from build123d import *

# Parameters (mm, degrees)
SKETCH1_W               = 25.4
SKETCH1_H               = 25.4
BOSS_EXTRUDE1_DEPTH     = 5
F_1_4_CLEARANCE_HOLE1_D = 6.7564
SKETCH4_R               = 1.75
SKETCH4_W               = 25.4
SKETCH4_H               = 5
BOSS_EXTRUDE2_DEPTH     = 3
FILLET1_R               = 6


with BuildPart() as part:
    # Sketch1 → Boss-Extrude1 (new body)
    with BuildSketch(Plane(origin=(0, 0, 0), x_dir=(1, 0, 0), z_dir=(0, 1, 0))):
        Rectangle(SKETCH1_W, SKETCH1_H)
    extrude(amount=BOSS_EXTRUDE1_DEPTH)

    # 1/4 Clearance Hole1 (through all)
    with Locations(Plane(origin=(0, 5, 0), x_dir=(1, 0, 0), z_dir=(0, 1, 0))):
        with Locations((0, 0)):
            Hole(F_1_4_CLEARANCE_HOLE1_D / 2)

    # Sketch4 → Boss-Extrude2 (add, symmetric)
    # profile 1 of 2: a face of its own
    with BuildSketch(Plane.XY.offset(12.7)):
        Polygon((-35, 5), (-35, -56), (35, -56), (35, 5), (12.7, 5), (12.7, 0), (-12.7, 0), (-12.7, 5), align=None)
        with Locations((-29, -50)):
            Circle(SKETCH4_R, mode=Mode.SUBTRACT)
        with Locations((29, -50)):
            Circle(SKETCH4_R, mode=Mode.SUBTRACT)
        with Locations((-29, -1)):
            Circle(SKETCH4_R, mode=Mode.SUBTRACT)
        with Locations((29, -1)):
            Circle(SKETCH4_R, mode=Mode.SUBTRACT)
    # profile 2 of 2: a face of its own
    with BuildSketch(Plane.XY.offset(12.7)):
        with Locations((0, 2.5)):
            Rectangle(SKETCH4_W, SKETCH4_H)
    extrude(amount=BOSS_EXTRUDE2_DEPTH, both=True)

    # Fillet1
    fillet1_edges = [part.edges().sort_by_distance(p)[0] for p in [
        (-35, 5, 12.7),
        (35, 5, 12.7),
        (35, -56, 12.7),
        (-35, -56, 12.7),
    ]]
    fillet(fillet1_edges, radius=FILLET1_R)


solid = part.part
Input: part model. Units: mm. Frame: model coordinates. A direction names the side the tool comes from. Coordinates: 2 decimals unless noted, no trailing zeros. Loops run counter-clockwise (first coordinate to the right, second up) from the corner with the lowest first, then second, coordinate; pieces in that order, holes last.
Q1. Cut plane D-D (y = -38). Output: boundary loops of the cut face in (x, z).
Q2. Draft query along Y for faces 1 (the face through (-30.75, -0.92, 12.66)), 2 (the face through (33.289, -54.196, 12.658)), 3 (the face through (0, 2, -12.7)). Return one class per face: +Y half, -Y half, draft (parallel to the pull), parting line (faces both ways), or undercut.
Q3. Material intervals for line 1 (Y direction, x = -29, z = 12.85); line 2 (Z direction, x = 26, y = -16); line 3 (Y direction, x = -3, z = -4.75), sorted ascending.
Q4. Contact query for flat-ended pins moving along their axis: pin 1 (5.5 mm diameter, centred on x = 29, y = -50, fed in from -Z); pin 2 (4 mm diameter, centred on y = 1.5, z = 1, fed in from -X); pin 3 (1.5 mm diameter, centred on y = 1.5, z = -3.5, fed in from +X). Output: stop coordinate, or through.
Q5. Cut plane B-B (z = 13). Output: boundary loops of the cut face in (x, y), then the cut area to 3 significant figures.
Q6. Set-up query: faces 4 (the face through (33.196, 3.289, 12.658)), 5 (the face through (12.7, 2, -1)), 6 (the face through (-12.7, 2, -1)). Return all of +Z, -Z, +X, -X, +Y, -Y with unobstructed straight access to the full face (end or side cutting, diameter ignored); none if empty.
Q7. Cut plane A-A (z = 0). Output: boundary loops of the cut face in (x, y), then the cut area to 3 significant figures.
Q8. Cut plane C-C (x = 5). Output: boundary loops of the cut face in (y, z), then the cut area to 3 significant figures.
Working result:
1. outline: (-35, 9.7) - (35, 9.7) - (35, 15.7) - (-35, 15.7) - close
2. face 1: undercut
2. face 2: -Y half
2. face 3: draft
3. line 1: y = -56 to -51.75, -48.25 to -2.75, 0.75 to 5
3. line 2: z = 9.7 to 15.7
3. line 3: y = 0 to 5
4. pin 1: stops at z = 9.7
4. pin 2: stops at x = -12.7
4. pin 3: stops at x = 12.7
5. outline: (-35, -50) arc R6 ccw to (-29, -56) - (29, -56) arc R6 ccw to (35, -50) - (35, -1) arc R6 ccw to (29, 5) - (-29, 5) arc R6 ccw to (-35, -1) - close; hole circle Ø3.5 at (-29, -50); hole circle Ø3.5 at (-29, -1); hole circle Ø3.5 at (29, -50); hole circle Ø3.5 at (29, -1)
5. area: 4,200 mm2
6. face 4: +Z, -Z, +X, +Y
6. face 5: -Z, +X, +Y, -Y
6. face 6: -Z, -X, +Y, -Y
7. outline: (-12.7, 0) - (-3.38, 0) - (-3.38, 5) - (-12.7, 5) - close; (3.38, 0) - (12.7, 0) - (12.7, 5) - (3.38, 5) - close
7. area: 93.2 mm2
8. outline: (-56, 9.7) - (0, 9.7) - (0, -12.7) - (5, -12.7) - (5, 15.7) - (-56, 15.7) - close
8. area: 478 mm2
